Check sheet for the modelled part. Datum: model origin and axes. Units: mm. Give positions to 0.01 mm unless a question says otherwise; leave off trailing zeros. Order: outer loops, then holes, each group sorted by start corner. A loop starts at its lowest first (then second) coordinate and runs counter-clockwise, first axis right, second up.
from build123d import *

# Parameters (mm, degrees)
SKETCH1_W                = 130
SKETCH1_H                = 130
BOSS_EXTRUDE1_DEPTH      = 3
FILLET1_R                = 5
SKETCH2_R                = 4.75
CUT_EXTRUDE1_DEPTH       = 92.972822073
F_5_0_5_DIAMETER_HOLE1_D = 5
F_4_0_4_DIAMETER_HOLE1_D = 4
SKETCH8_R                = 10
CUT_EXTRUDE2_DEPTH       = 92.972822073
F_4_0_4_DIAMETER_HOLE2_D = 4


with BuildPart() as part:
    # Sketch1 → Boss-Extrude1 (new body)
    with BuildSketch(Plane(origin=(0, 0, 0), x_dir=(1, 0, 0), z_dir=(0, 1, 0))):
        Rectangle(SKETCH1_W, SKETCH1_H)
    extrude(amount=BOSS_EXTRUDE1_DEPTH)

    # Fillet1
    fillet1_edges = [part.edges().sort_by_distance(p)[0] for p in [
        (65, 1.5, 65),
        (-65, 1.5, 65),
        (-65, 1.5, -65),
        (65, 1.5, -65),
    ]]
    fillet(fillet1_edges, radius=FILLET1_R)

    # Sketch2 → Cut-Extrude1 (cut, through all)
    with BuildSketch(Plane(origin=(0, 0, 0), x_dir=(1, 0, 0), z_dir=(0, 1, 0))):
        with Locations(Location((0, 0, 0), (0, 0, 270))):
            Circle(SKETCH2_R)
    extrude(amount=CUT_EXTRUDE1_DEPTH, mode=Mode.SUBTRACT)

    # Ø5.0 (5) Diameter Hole1 (through all)
    with Locations(Plane(origin=(0, 0, 0), x_dir=(-1, 0, 0), z_dir=(0, -1, 0))):
        with Locations((60.313708499, 11.313708499), (60.313708499, -11.313708499), (37.686291501, -11.313708499), (37.686291501, 11.313708499)):
            f_5_0_5_diameter_hole1 = Hole(F_5_0_5_DIAMETER_HOLE1_D / 2)

    # Mirror1: Ø5.0 (5) Diameter Hole1 across plane
    add(f_5_0_5_diameter_hole1.mirror(Plane(origin=(0, 0, 0), x_dir=(0, 0, 1), z_dir=(1, 0, 0))), mode=Mode.SUBTRACT)

    # Ø4.0 (4) Diameter Hole1 (through all)
    with Locations(Plane(origin=(0, 3, 0), x_dir=(1, 0, 0), z_dir=(0, 1, 0))):
        with Locations((38, 51), (-38, 51)):
            Hole(F_4_0_4_DIAMETER_HOLE1_D / 2)

    # Sketch8 → Cut-Extrude2 (cut, through all)
    with BuildSketch(Plane(origin=(0, 0, 0), x_dir=(1, 0, 0), z_dir=(0, 1, 0))):
        with Locations(Location((0, -49, 0), (0, 0, 270))):
            Circle(SKETCH8_R)
        with BuildLine():
            Line((10.75, -35), (10.75, -10))
            ThreePointArc((10.75, -10), (13, -7.75), (15.25, -10))
            Line((15.25, -10), (15.25, -35))
            ThreePointArc((15.25, -35), (13, -37.25), (10.75, -35))
        make_face()
        with BuildLine():
            Line((-10.75, -35), (-10.75, -10))
            ThreePointArc((-10.75, -10), (-13, -7.75), (-15.25, -10))
            Line((-15.25, -10), (-15.25, -35))
            ThreePointArc((-15.25, -35), (-13, -37.25), (-10.75, -35))
        make_face()
    extrude(amount=CUT_EXTRUDE2_DEPTH, mode=Mode.SUBTRACT)

    # Ø4.0 (4) Diameter Hole2 (through all)
    with Locations(Plane(origin=(0, 3, 0), x_dir=(1, 0, 0), z_dir=(0, 1, 0))):
        with Locations((-15, -54.25), (-15, -43.75)):
            Hole(F_4_0_4_DIAMETER_HOLE2_D / 2)


solid = part.part
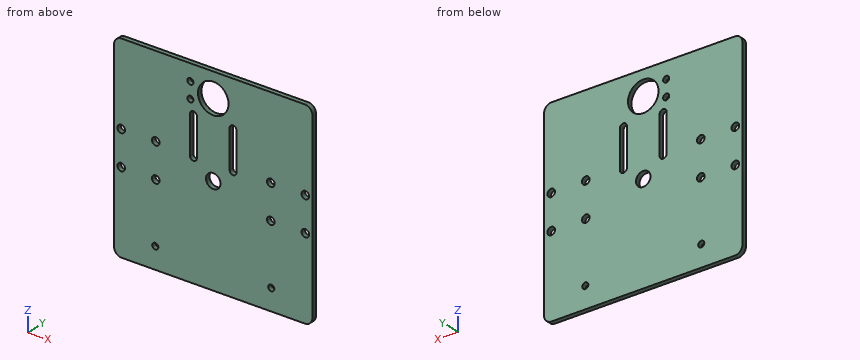
1) Section check B-B, the plane z = 54.25. Record the cut outline in (x, y), then the cut area to 3 significant figures.
Recorded:
outline: (-65, 0) - (-17, 0) - (-17, 3) - (-65, 3) - close; (-13, 0) - (-8.51, 0) - (-8.51, 3) - (-13, 3) - close; (8.51, 0) - (65, 0) - (65, 3) - (8.51, 3) - close
area: 327 mm2
2) Material ranges on L1, parallel to Z at x = -15, y = 2.25; L2, parallel to X at y = 1.95, z = 0; L3, parallel to X at y = 2.35, z = 52.5, recorded low to high.
Recorded:
L1: z = -65 to 8.97, 36.03 to 41.75, 45.75 to 52.25, 56.25 to 65
L2: x = -65 to -4.75, 4.75 to 65
L3: x = -65 to -15.97, -14.03 to -9.37, 9.37 to 65
3) Section check C-C, the plane y = 1.2. State how many separate pieces and enclosed holes the cut face has, then the cut area to 3 significant figures.
Recorded:
separate pieces: 1
enclosed holes: 16
area: 16,000 mm2
4) Section check A-A, the plane x = 0. Record the cut outline in (y, z), then the cut area to 4 significant figures.
Recorded:
outline: (0, -65) - (3, -65) - (3, -4.75) - (0, -4.75) - close; (0, 4.75) - (3, 4.75) - (3, 39) - (0, 39) - close; (0, 59) - (3, 59) - (3, 65) - (0, 65) - close
area: 301.5 mm2
5) Section check D-D, the plane x = 38. Record the cut outline in (y, z), then the cut area to 3 significant figures.
Recorded:
outline: (0, -65) - (3, -65) - (3, -53) - (0, -53) - close; (0, -49) - (3, -49) - (3, -13.79) - (0, -13.79) - close; (0, -8.83) - (3, -8.83) - (3, 8.83) - (0, 8.83) - close; (0, 13.79) - (3, 13.79) - (3, 65) - (0, 65) - close
area: 348 mm2
